Geometry check sheet. Reference: the model listing, model coordinates, mm. Face numbers are marked on the shaded views. Coordinates: 2 decimals unless noted, no trailing zeros. Order: outer loops, then holes, each group sorted by start corner. A loop starts at its lowest first (then second) coordinate and runs counter-clockwise, first axis right, second up. Notation, with made-up numbers: M -30,36 L -25,36 A8 ccw -25,48 Z; hole C 34,15.5 d3. An arc over 180 degrees is marked long. One line per item, written item: value. Start each with the question number.
1) Draft check along Z on the marked faces 1, 2 and 3. Enter one of: pulls with the +Z half, pulls with the -Z half, needs draft (parallel to the pull), parting line crosses it, or undercut.
2) Thickness scan on L1, parallel to Z at x = -434, y = -99.5; L2, parallel to Y at x = 0, z = -0.8; L3, parallel to Y at x = 546, z = -248.5. Record the ranges inside material, lowest first. Write a range as from..to.
3) Sectioned sample at B-B, the plane z = -282. Enter the section's corners in (x, y).
4) Go/stop test with flat-tipped pins: P1, Ø1.6, axis at x = -200.5, z = -369, coming from the +Y side; P2, Ø1.5, axis at x = 764.5, y = -31.5, coming from the +Z side; P3, Ø6, axis at x = 1, z = -195.5, coming from the +Y side. Record where each tip stops, or that it passes through.
5) Sectioned sample at A-A, the plane x = -508. Enter the section's corners in (y, z).
```python
from build123d import *

# Parameters (mm, degrees)
BASE_FLANGE1_DEPTH = 1150
SKETCH2_R          = 15
CUT_EXTRUDE1_DEPTH = 10


# Sheet-metal steps are written as plain solids
with BuildPart() as part:
    # Sketch1 → Base-Flange1 (new, symmetric)
    with BuildSketch(Plane(origin=(0, 0, 0), x_dir=(0, 0, -1), z_dir=(1, 0, 0))):
        with BuildLine():
            Line((0, 0), (0, -145.5))
            ThreePointArc((0, -145.5), (1.318019485, -148.681980515), (4.5, -150))
            Line((4.5, -150), (365.5, -150))
            ThreePointArc((365.5, -150), (368.681980515, -148.681980515), (370, -145.5))
            Line((370, -145.5), (370, -50))
            Line((370, -50), (368, -50))
            Line((368, -50), (368, -145.5))
            ThreePointArc((368, -145.5), (367.267766953, -147.267766953), (365.5, -148))
            Line((365.5, -148), (4.5, -148))
            ThreePointArc((4.5, -148), (2.732233047, -147.267766953), (2, -145.5))
            Line((2, -145.5), (2, 0))
            Line((2, 0), (0, 0))
        make_face()
    extrude(amount=BASE_FLANGE1_DEPTH, both=True)

    # Sketch2 → Cut-Extrude1 (cut)
    with BuildSketch(Plane.XY):
        with Locations((0, -115)):
            Circle(SKETCH2_R)
    extrude(amount=-CUT_EXTRUDE1_DEPTH, mode=Mode.SUBTRACT)


solid = part.part
```
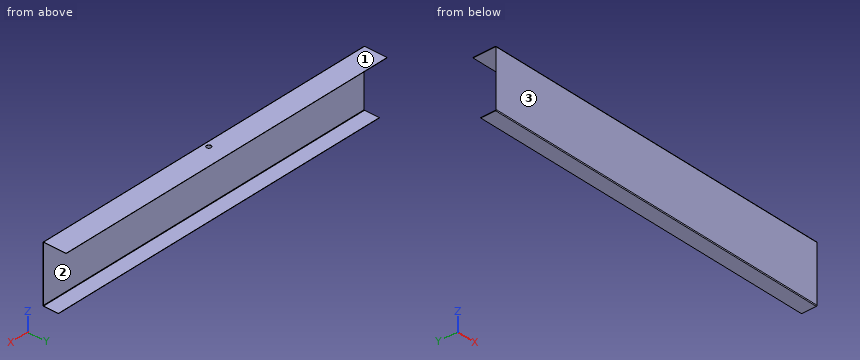
Final values:
1. face 1: pulls with the +Z half
1. face 2: undercut
1. face 3: needs draft
2. L1: z = -370..-368, -2..0
2. L2: y = -148.06..-130, -100..0
2. L3: y = -150..-148
3. outline: M -1150,-150 L 1150,-150 L 1150,-148 L -1150,-148 Z
4. P1: stops at y = -50
4. P2: stops at z = 0
4. P3: stops at y = -148
5. outline: M -150,-365.5 A4.5 ccw -145.5,-370 L -50,-370 L -50,-368 L -145.5,-368 A2.5 cw -148,-365.5 L -148,-4.5 A2.5 cw -145.5,-2 L 0,-2 L 0,0 L -145.5,0 A4.5 ccw -150,-4.5 Z
